Answer from the drawing. Dimensions are ordinates in mm from the lowest x, y and z of the part. Round coordinates to 2 decimals unless told otherwise and drop trailing zeros. Loops run counter-clockwise (first coordinate to the right, second up) from the corner with the lowest first, then second, coordinate; pieces in that order, holes last. Notation, with made-up numbers: M -4,25.25 L 25,25.25 A31 ccw 25,60.25 Z; hole C -33,-19.75 d10. An arc over 180 degrees is marked long. One line per item, written item: value.
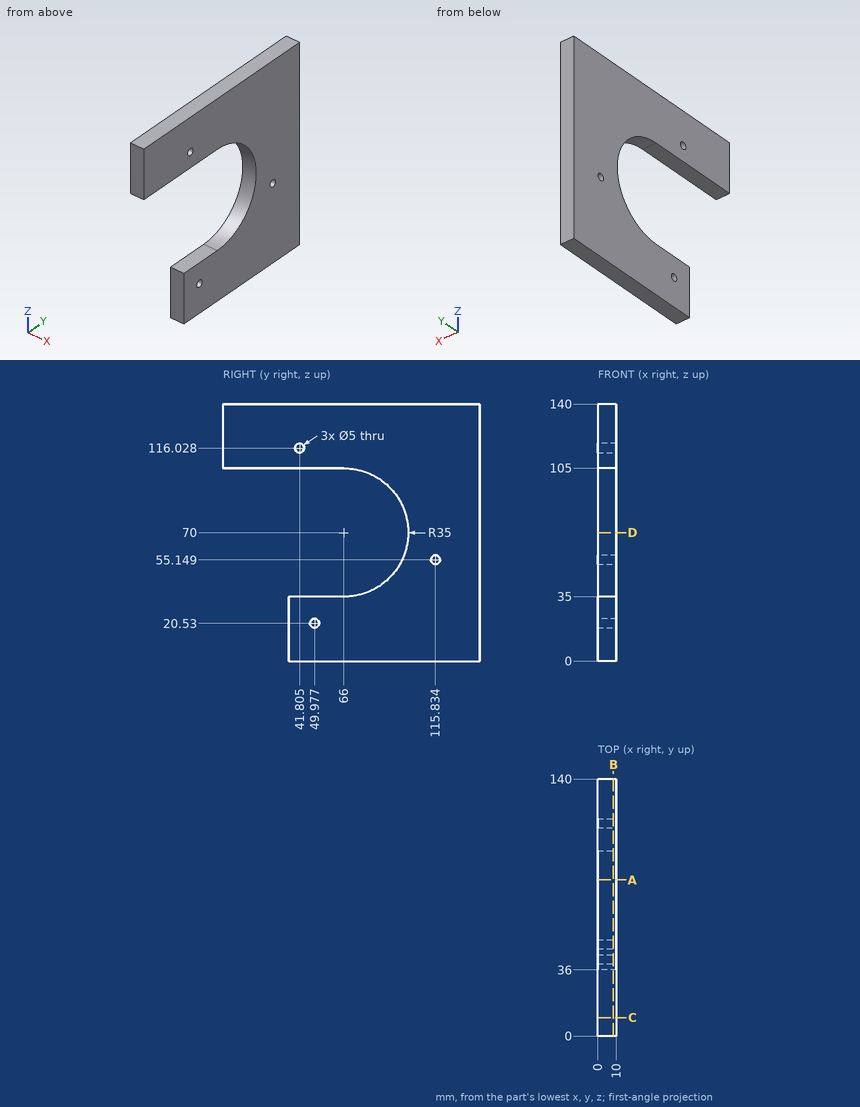
1) Find section A-A (y = 85). Give the vertices of the cut face in (x, z), then the cut area to 3 significant figures.
Check values:
outline: M 0,0 L 10,0 L 10,40.61 L 0,40.61 Z; M 0,99.39 L 10,99.39 L 10,140 L 0,140 Z
area: 812 mm2
2) Each of these flat-tipped pins is pushed along its axis until it touches: pin 1 (3 mm diameter, centred on x = 6, y = 32.5, fed in from -Z); pin 2 (4 mm diameter, centred on x = 7.5, y = 42, fed in from -Z); pin 3 (4 mm diameter, centred on y = 115.83, z = 55.15, fed in from +X); pin 4 (5 mm diameter, centred on x = 6.5, z = 11, fed in from -Y). Where does it stop, or does it pass through?
Check values:
pin 1: z = 105
pin 2: z = 0
pin 3: through
pin 4: y = 36
3) Find section B-B (x = 8.5). Give the vertices of the cut face in (y, z) (1 decimal).
Check values:
outline: M 0,105 L 66,105 A35 cw 66,35 L 36,35 L 36,0 L 140,0 L 140,140 L 0,140 Z; hole C 41.8,116 d5; hole C 50,20.5 d5; hole C 115.8,55.1 d5
4) Find section D-D (z = 70). Give the vertices of the cut face in (x, y), then the cut area to 3 significant figures.
Check values:
outline: M 0,101 L 10,101 L 10,140 L 0,140 Z
area: 390 mm2
5) Find section C-C (y = 10). Give the vertices of the cut face in (x, z), then the cut area to 3 significant figures.
Check values:
outline: M 0,105 L 10,105 L 10,140 L 0,140 Z
area: 350 mm2
6) Find the intervals of material crossed by probe 1 along Z at (x, y) = (2.5, 83) (1 decimal); probe 2 along Z at (x, y) = (4, 39.5) (1 decimal); probe 3 along Z at (x, y) = (3.25, 96), in increasing order. Write a range as from..to.
Check values:
probe 1: 0..39.4, 100.6..140
probe 2: 0..35, 105..115.1, 117..140
probe 3: 0..51.97, 88.03..140
